Here's how the part is built. I have some questions about the finished solid (model axes, mm). A direction names the side the tool comes from. Coordinates: 2 decimals unless noted, no trailing zeros. Write each loop counter-clockwise with the first axis right and the second up, starting at its lowest first coordinate (ties: lowest second). Pieces come first, ordered by that corner, then holes.
(1) Imagine slicing it at A-A, the plane x = 68.5. List the corners of the cut face in (y, z) for me.
(2) Imagine slicing it at B-B, the plane z = 10. List the corners of the cut face in (x, y) for me, plus the area to 3 significant figures.
(3) Imagine slicing it at C-C, the plane x = 100.5. List the corners of the cut face in (y, z) for me.
(4) For pin 1 Ø13.5 at (x, y) = (139.7, 19.74) entering from -Z, with a flat end and sliding along its axis, tell me the tip position at first contact or that it passes through.
(5) Please list where these lines run through material, in increasing order: probe 1 along X at (y, z) = (-33, 24.25); probe 2 along X at (y, z) = (-68, 8.25); probe 3 along Y at (x, z) = (108, 14.75).
(6) Thinking about a two-plate mould opening in X: for faces 1 (the flat face through (-101, -94.56, 13)), 2 (the flat face through (-2, -107.95, 13)), 3 (the cylindrical face through (151.53, 100.31, 12.52)), 4 (the flat face through (114.3, -57, 13)), which applies, released by +X, released by -X, zero draft, split by the parting line, or undercut?
(7) Which directions (+Z, -Z, +X, -X, +Y, -Y) give clear straight access to the entire face, cutting with the end or side of a thin tool? Please do faces 5 (the flat face through (31.75, -70, 13)), 6 (the cylindrical face through (-151.135, 100.707, 12.522)).
```python
from build123d import *

# Parameters (mm, degrees)
SKETCH1_R                      = 11.422
BOSS_EXTRUDE1_DEPTH            = 25.4
SKETCH2_W                      = 50.8
SKETCH2_H                      = 25.4
FOAM_INSERT_CUT_THROUGHS_DEPTH = 25.4
SKETCH3_W                      = 25.4
SKETCH3_H                      = 76.2
CUT_EXTRUDE1_DEPTH             = 25.4


with BuildPart() as part:
    # Sketch1 → Boss-Extrude1 (new body)
    with BuildSketch(Plane.XY):
        with BuildLine():
            Line((-133.373251541, -107.95), (133.373251541, -107.95))
            ThreePointArc((133.373251541, -107.95), (151.333763783, -100.510512242), (158.773251541, -82.55))
            Line((158.773251541, -82.55), (158.773251541, 82.55))
            ThreePointArc((158.773251541, 82.55), (151.333763783, 100.510512242), (133.373251541, 107.95))
            Line((133.373251541, 107.95), (-133.373251541, 107.95))
            ThreePointArc((-133.373251541, 107.95), (-151.333763783, 100.510512242), (-158.773251541, 82.55))
            Line((-158.773251541, 82.55), (-158.773251541, -82.55))
            ThreePointArc((-158.773251541, -82.55), (-151.333763783, -100.510512242), (-133.373251541, -107.95))
        make_face()
        with Locations((-139.7, 19.739923182)):
            Circle(SKETCH1_R, mode=Mode.SUBTRACT)
        with Locations((139.7, 19.739923182)):
            Circle(SKETCH1_R, mode=Mode.SUBTRACT)
    extrude(amount=BOSS_EXTRUDE1_DEPTH)

    # Sketch2 → Foam Insert Cut-Throughs (cut)
    with BuildSketch(Plane(origin=(0, 0, 0), x_dir=(-1, 0, 0), z_dir=(0, 0, -1))):
        with Locations((-57.15, -69.85)):
            Rectangle(SKETCH2_W, SKETCH2_H)
        with Locations((57.15, -69.85)):
            Rectangle(SKETCH2_W, SKETCH2_H)
    extrude(amount=-FOAM_INSERT_CUT_THROUGHS_DEPTH, mode=Mode.SUBTRACT)

    # Sketch3 → Cut-Extrude1 (cut)
    with BuildSketch(Plane(origin=(0, 0, 0), x_dir=(-1, 0, 0), z_dir=(0, 0, -1))):
        with Locations((101.6, -56.460076818)):
            Rectangle(SKETCH3_W, SKETCH3_H)
        with Locations((-101.6, -56.460076818)):
            Rectangle(SKETCH3_W, SKETCH3_H)
    extrude(amount=-CUT_EXTRUDE1_DEPTH, mode=Mode.SUBTRACT)


solid = part.part
```
Recorded:
1. outline: (-107.95, 0) - (-82.55, 0) - (-82.55, 25.4) - (-107.95, 25.4) - close; (-57.15, 0) - (107.95, 0) - (107.95, 25.4) - (-57.15, 25.4) - close
2. outline: (-158.77, -82.55) arc R25.4 ccw to (-133.37, -107.95) - (133.37, -107.95) arc R25.4 ccw to (158.77, -82.55) - (158.77, 82.55) arc R25.4 ccw to (133.37, 107.95) - (-133.37, 107.95) arc R25.4 ccw to (-158.77, 82.55) - close; hole circle Ø22.84 at (-139.7, 19.74); hole (-114.3, -94.56) - (-88.9, -94.56) - (-88.9, -18.36) - (-114.3, -18.36) - close; hole (-82.55, -82.55) - (-31.75, -82.55) - (-31.75, -57.15) - (-82.55, -57.15) - close; hole (31.75, -82.55) - (82.55, -82.55) - (82.55, -57.15) - (31.75, -57.15) - close; hole (88.9, -94.56) - (114.3, -94.56) - (114.3, -18.36) - (88.9, -18.36) - close; hole circle Ø22.84 at (139.7, 19.74)
2. area: 60,700 mm2
3. outline: (-107.95, 0) - (-94.56, 0) - (-94.56, 25.4) - (-107.95, 25.4) - close; (-18.36, 0) - (107.95, 0) - (107.95, 25.4) - (-18.36, 25.4) - close
4. pin 1: passes through
5. probe 1: x = -158.77 to -114.3, -88.9 to 88.9, 114.3 to 158.77
5. probe 2: x = -158.77 to -114.3, -88.9 to -82.55, -31.75 to 31.75, 82.55 to 88.9, 114.3 to 158.77
5. probe 3: y = -107.95 to -94.56, -18.36 to 107.95
6. face 1: undercut
6. face 2: zero draft
6. face 3: released by +X
6. face 4: undercut
7. face 5: +Z, -Z
7. face 6: +Z, -Z, -X, +Y
